from build123d import *

# Parameters (mm, degrees)
Y_KSEKLIK_EKSTR_ZYON1_DEPTH = 20
CUT_EXTRUDE1_DEPTH          = 44
CUT_EXTRUDE1_DEPTH_BACK     = 10
SKETCH1_R                   = 2.5
SKETCH2_W                   = 32
SKETCH2_H                   = 30
CUT_EXTRUDE3_DEPTH          = 27
SKETCH3_W                   = 32
SKETCH3_H                   = 30
BOSS_EXTRUDE1_DEPTH         = 16
CUT_EXTRUDE4_DEPTH          = 4
SKETCH5_W                   = 33.515954684
SKETCH5_H                   = 18.308274805
BOSS_EXTRUDE2_DEPTH         = 10
CUT_EXTRUDE5_DEPTH          = 53
CUT_EXTRUDE5_DEPTH_BACK     = 25
SKETCH6_R                   = 2.5
SKETCH7_W                   = 36.495036791
SKETCH7_H                   = 91.485439351
SKETCH7_W_2                 = 38.306268879
CUT_EXTRUDE7_DEPTH          = 30
SKETCH8_W                   = 29
SKETCH8_H                   = 90
BOSS_EXTRUDE3_DEPTH         = 10
CUT_EXTRUDE8_DEPTH          = 10
SKETCH10_W                  = 32
SKETCH10_H                  = 30
CUT_EXTRUDE9_DEPTH          = 28
SKETCH11_W                  = 32
SKETCH11_H                  = 30
BOSS_EXTRUDE4_DEPTH         = 10
SKETCH12_R                  = 3
CUT_EXTRUDE10_DEPTH         = 22
SKETCH13_R                  = 6
CUT_EXTRUDE11_DEPTH         = 5


with BuildPart() as part:
    # Çizim1 → Yükseklik-Ekstrüzyon1 (new body)
    with BuildSketch(Plane.XY):
        with BuildLine():
            Line((-41.541366964, -1.110887656), (-41.541366964, 48.889112344))
            ThreePointArc((-41.541366964, 48.889112344), (-35.683502588, 63.031247968), (-21.541366964, 68.889112344))
            Line((-21.541366964, 68.889112344), (28.458633036, 68.889112344))
            ThreePointArc((28.458633036, 68.889112344), (42.600768659, 63.031247968), (48.458633036, 48.889112344))
            Line((48.458633036, 48.889112344), (48.458633036, -1.110887656))
            ThreePointArc((48.458633036, -1.110887656), (42.600768659, -15.25302328), (28.458633036, -21.110887656))
            Line((28.458633036, -21.110887656), (-21.541366964, -21.110887656))
            ThreePointArc((-21.541366964, -21.110887656), (-35.683502588, -15.25302328), (-41.541366964, -1.110887656))
        make_face()
    extrude(amount=Y_KSEKLIK_EKSTR_ZYON1_DEPTH)

    # Sketch1 → Cut-Extrude1 (cut, two sides: drawn at the far end of the back side and taken through both)
    with BuildSketch(Plane.XY.offset(-CUT_EXTRUDE1_DEPTH_BACK)):
        with Locations(Location((-4.041366964, 23.889112344, 0), (0, 0, 180))):
            Circle(SKETCH1_R)
        with Locations(Location((10.958633036, 23.889112344, 0), (0, 0, 180))):
            Circle(SKETCH1_R)
    extrude(amount=CUT_EXTRUDE1_DEPTH + CUT_EXTRUDE1_DEPTH_BACK, mode=Mode.SUBTRACT)

    # Sketch2 → Cut-Extrude3 (cut)
    with BuildSketch(Plane.XY):
        with Locations((3.458633036, 53.889112344)):
            Rectangle(SKETCH2_W, SKETCH2_H)
    extrude(amount=CUT_EXTRUDE3_DEPTH, mode=Mode.SUBTRACT)

    # Sketch3 → Boss-Extrude1 (add)
    with BuildSketch(Plane.XY):
        with Locations((3.458633036, 53.889112344)):
            Rectangle(SKETCH3_W, SKETCH3_H)
    extrude(amount=BOSS_EXTRUDE1_DEPTH)

    # Sketch4 → Cut-Extrude4 (cut)
    with BuildSketch(Plane.XY):
        Polygon((15.692905243, 23.889112344), (13.325769139, 27.989112344), (8.591496932, 27.989112344), (6.224360828, 23.889112344), (8.591496932, 19.789112344), (13.325769139, 19.789112344), align=None)
        Polygon((0.692905243, 23.889112344), (-1.674230861, 27.989112344), (-6.408503068, 27.989112344), (-8.775639172, 23.889112344), (-6.408503068, 19.789112344), (-1.674230861, 19.789112344), align=None)
    extrude(amount=CUT_EXTRUDE4_DEPTH, mode=Mode.SUBTRACT)

    # Sketch5 → Boss-Extrude2 (add)
    with BuildSketch(Plane.XY):
        with Locations((2.203630327, 23.667641278)):
            Rectangle(SKETCH5_W, SKETCH5_H)
    extrude(amount=BOSS_EXTRUDE2_DEPTH)

    # Sketch6 → Cut-Extrude5 (cut, two sides: drawn at the far end of the back side and taken through both)
    with BuildSketch(Plane.XY.offset(-CUT_EXTRUDE5_DEPTH_BACK)):
        with Locations(Location((-4.041366964, 23.889112344, 0), (0, 0, 180))):
            Circle(SKETCH6_R)
        with Locations(Location((10.958633036, 23.889112344, 0), (0, 0, 180))):
            Circle(SKETCH6_R)
    extrude(amount=CUT_EXTRUDE5_DEPTH + CUT_EXTRUDE5_DEPTH_BACK, mode=Mode.SUBTRACT)

    # Sketch7 → Cut-Extrude7 (cut)
    with BuildSketch(Plane.XY):
        with Locations((-30.78888536, 23.146392668)):
            Rectangle(SKETCH7_W, SKETCH7_H)
        with Locations((38.611767476, 23.146392668)):
            Rectangle(SKETCH7_W_2, SKETCH7_H)
    extrude(amount=CUT_EXTRUDE7_DEPTH, mode=Mode.SUBTRACT)

    # Sketch8 → Boss-Extrude3 (add)
    with BuildSketch(Plane.XY):
        with Locations((-27.041366964, 23.889112344)):
            Rectangle(SKETCH8_W, SKETCH8_H)
        with Locations((33.958633036, 23.889112344)):
            Rectangle(SKETCH8_W, SKETCH8_H)
    extrude(amount=BOSS_EXTRUDE3_DEPTH)

    # Sketch9 → Cut-Extrude8 (cut)
    with BuildSketch(Plane.XY):
        with BuildLine():
            Line((-41.541366964, 68.889112344), (-21.541366964, 68.889112344))
            ThreePointArc((-21.541366964, 68.889112344), (-35.683502588, 63.031247968), (-41.541366964, 48.889112344))
            Line((-41.541366964, 48.889112344), (-41.541366964, 68.889112344))
        make_face()
        with BuildLine():
            Line((48.458633036, 68.889112344), (48.458633036, 48.889112344))
            ThreePointArc((48.458633036, 48.889112344), (42.600768659, 63.031247968), (28.458633036, 68.889112344))
            Line((28.458633036, 68.889112344), (48.458633036, 68.889112344))
        make_face()
        with BuildLine():
            Line((48.458633036, -21.110887656), (28.458633036, -21.110887656))
            ThreePointArc((28.458633036, -21.110887656), (42.600768659, -15.25302328), (48.458633036, -1.110887656))
            Line((48.458633036, -1.110887656), (48.458633036, -21.110887656))
        make_face()
        with BuildLine():
            Line((-41.541366964, -21.110887656), (-41.541366964, -1.110887656))
            ThreePointArc((-41.541366964, -1.110887656), (-35.683502588, -15.25302328), (-21.541366964, -21.110887656))
            Line((-21.541366964, -21.110887656), (-41.541366964, -21.110887656))
        make_face()
    extrude(amount=CUT_EXTRUDE8_DEPTH, mode=Mode.SUBTRACT)

    # Sketch10 → Cut-Extrude9 (cut)
    with BuildSketch(Plane.XY):
        with Locations((3.458633036, 53.889112344)):
            Rectangle(SKETCH10_W, SKETCH10_H)
        with Locations((3.458633036, -6.110887656)):
            Rectangle(SKETCH10_W, SKETCH10_H)
    extrude(amount=CUT_EXTRUDE9_DEPTH, mode=Mode.SUBTRACT)

    # Sketch11 → Boss-Extrude4 (add)
    with BuildSketch(Plane.XY):
        with Locations((3.458633036, 53.889112344)):
            Rectangle(SKETCH11_W, SKETCH11_H)
        with Locations((3.458633036, -6.110887656)):
            Rectangle(SKETCH11_W, SKETCH11_H)
    extrude(amount=BOSS_EXTRUDE4_DEPTH)

    # Sketch12 → Cut-Extrude10 (cut)
    with BuildSketch(Plane.XY):
        with Locations(Location((-4.041366964, 23.889112344, 0), (0, 0, 180))):
            Circle(SKETCH12_R)
        with Locations(Location((10.958633036, 23.889112344, 0), (0, 0, 180))):
            Circle(SKETCH12_R)
    extrude(amount=CUT_EXTRUDE10_DEPTH, mode=Mode.SUBTRACT)

    # Sketch13 → Cut-Extrude11 (cut)
    with BuildSketch(Plane.XY):
        with Locations((10.958633036, 23.889112344)):
            Circle(SKETCH13_R)
        with Locations((-4.041366964, 23.889112344)):
            Circle(SKETCH13_R)
    extrude(amount=CUT_EXTRUDE11_DEPTH, mode=Mode.SUBTRACT)


solid = part.part
Input: part model. Units: mm. Frame: model coordinates. A direction names the side the tool comes from. Round coordinates to 2 decimals unless told otherwise and drop trailing zeros. Loops run counter-clockwise (first coordinate to the right, second up) from the corner with the lowest first, then second, coordinate; pieces in that order, holes last. Notation, with made-up numbers: M 37.25,63 L 93.25,63 A12 cw 93.25,68 Z; hole C -8.5,87 d10. An arc over 180 degrees is marked long. Answer as CSV lines item,"result". Start each with the question number.
(1) First-contact query: pin 1 (1 mm diameter, centred on x = 35.5, z = 7.5, fed in from +Y); pin 2 (6 mm diameter, centred on y = -9, z = 12, fed in from +X); pin 3 (2 mm diameter, centred on x = -27, z = 10, fed in from -Y). Flat tips, straight axial feed; report the tip coordinate or a pass-through.
(2) Section D-D, the plane x = 37. Output: boundary loops of the cut face in (y, z), plus the area to 3 significant figures.
(3) Section B-B, the plane x = 10.5. Output: boundary loops of the cut face in (y, z), plus the area to 3 significant figures.
(4) Reachability of faces 5 (the flat face through (19.459, 24, 15)), 6 (the flat face through (-12.541, 24, 15)), 7 (the cylindrical face through (9.66, 18.03, 2.46)), 8 (the flat face through (3, 38.889, 15)) from +Z, -Z, +X, -X, +Y, -Y: full face, straight path, thin tool, end or side. Return the list, or none.
(5) Section C-C, the plane y = 28.5. Output: boundary loops of the cut face in (x, z).
(6) Draft query along Y for faces 1 (the flat face through (12, 27, 5)), 2 (the flat face through (-3, 27, 5)), 3 (the cylindrical face through (-35.527, 63.186, 4.93)), 4 (the flat face through (48.459, 24, 5)). Return one class per face: released by +Y, released by -Y, zero draft, split by the parting line, or undercut.
(7) Line query: line 1 (X direction, y = 22, z = 16.75); line 2 (X direction, y = 27.5, z = 4.75); line 3 (Y direction, x = -3.5, z = 7.75). Output: solid intervals per line, ascending. Write a range as [from, to].
(8) Section A-A, the plane z = 3.5. Output: boundary loops of the cut face in (x, y).
Values found:
1,pin 1,"stops at y = 67.79"
1,pin 2,"stops at x = 47.64"
1,pin 3,"stops at y = -20.61"
2,outline,"M -19.2,0 L 66.97,0 L 66.97,10 L -19.2,10 Z"
2,area,"862 mm²"
3,outline,"M -21.11,0 L 17.91,0 L 17.91,5 L 20.92,5 L 20.92,20 L 8.89,20 L 8.89,10 L -21.11,10 Z; M 26.85,5 L 29.87,5 L 29.87,0 L 68.89,0 L 68.89,10 L 38.89,10 L 38.89,20 L 26.85,20 Z"
3,area,"1,050 mm²"
4,face 5,"+Z, +X, +Y, -Y"
4,face 6,"+Z, -X, +Y, -Y"
4,face 7,"-Z"
4,face 8,"+Z, +X, -X, +Y"
5,outline,"M -41.54,0 L -7.88,0 L -7.88,5 L -0.2,5 L -0.2,0 L 7.12,0 L 7.12,5 L 14.8,5 L 14.8,0 L 48.46,0 L 48.46,10 L 19.46,10 L 19.46,20 L -12.54,20 L -12.54,10 L -41.54,10 Z"
6,face 1,"undercut"
6,face 2,"undercut"
6,face 3,"released by +Y"
6,face 4,"zero draft"
7,line 1,"x = [-12.54, -6.37], [-1.71, 8.63], [13.29, 19.46]"
7,line 2,"x = [-41.54, -8.83], [0.75, 6.17], [15.75, 48.46]"
7,line 3,"y = [-21.11, 20.94], [26.84, 68.89]"
8,outline,"M -41.54,-1.11 A20 ccw -21.54,-21.11 L 28.46,-21.11 A20 ccw 48.46,-1.11 L 48.46,48.89 A20 ccw 28.46,68.89 L -21.54,68.89 A20 ccw -41.54,48.89 Z; hole C -4.04,23.89 d12; hole C 10.96,23.89 d12"
